Source: CAD feature listing. Evaluate the final solid. Frame: model axes, mm. A direction names the side the tool comes from. Round coordinates to 2 decimals unless told otherwise and drop trailing zeros. Loops run counter-clockwise (first coordinate to the right, second up) from the corner with the lowest first, then second, coordinate; pieces in that order, holes last.
(1) Mould query, pull axis X, two halves, no side actions, for faces 5 (the flat face through (17.635, -56, 0)), 6 (the cylindrical face through (-48.051, 12.783, 17.555)), 7 (the flat face through (-16, 28.78, 10)). Classes: pulls with the +X half, pulls with the -X half, needs draft (parallel to the pull), parting line crosses it, or undercut.
(2) Set-up query: faces 1 (the flat face through (-68.325, -38, 0)), 2 (the flat face through (-29, 23.82, 14)), 3 (the cylindrical face through (-59.61, 2.46, 0.05)), 4 (the flat face through (0.325, 26, 18)). Return all of +Z, -Z, +X, -X, +Y, -Y with unobstructed straight access to the full face (end or side cutting, diameter ignored); none if empty.
(3) First-contact query: pin 1 Ø17.5 at (x, y) = (-52.5, -55) entering from +Z; pin 2 Ø3 at (y, z) = (-63, 12) entering from -X (3 decimals); pin 3 Ø1.2 at (x, y) = (-38, 0.5) entering from +Z; pin 4 Ø13 at (x, y) = (-62.825, 0) entering from -Z. Flat tips, straight axial feed; report the tip coordinate or a pass-through.
(4) Material intervals for probe 1 along X at (y, z) = (0.5, 15.5); probe 2 along Y at (x, z) = (-10.5, 14.5); probe 3 along Z at (x, y) = (-48, 14), sorted ascending.
(5) Section D-D, the plane x = -14. Return the cut outline in (y, z).
(6) Section A-A, the plane y = -17.65. Return the cut outline in (x, z) (3 decimals), plus the area to 3 significant figures.
(7) Section C-C, the plane y = 20.78. Return the cut outline in (x, z) (3 decimals), plus the area to 3 significant figures.
(8) Section B-B, the plane z = 12. Return the cut outline in (x, y) (3 decimals), plus the area to 3 significant figures.
```python
from build123d import *

# Parameters (mm, degrees)
SALIENTE_EXTRUIR1_DEPTH    = 3.84
SALIENTE_EXTRUIR2_DEPTH    = 27.82
CROQUIS5_W                 = 19.2
CROQUIS5_H                 = 4.96
SALIENTE_EXTRUIR3_DEPTH    = 20.22
REDONDEO1_R                = 0.6
REDONDEO4_R                = 0.6
CROQUIS6_R                 = 2.36
CORTAR_EXTRUIR1_DEPTH      = 53.95
SALIENTE_EXTRUIR6_DEPTH    = 27.82
CORTAR_EXTRUIR9_DEPTH      = 53
CORTAR_EXTRUIR9_DEPTH_BACK = 66
CROQUIS10_R                = 2.36
REDONDEO5_R                = 5
REDONDEO6_R                = 5
CROQUIS12_R                = 4.05
CORTAR_EXTRUIR10_DEPTH     = 15
REDONDEO8_R                = 2
REDONDEO9_R                = 1
REDONDEO10_R               = 1
REDONDEO12_R               = 2
REDONDEO13_R               = 1
REDONDEO14_R               = 1
REDONDEO15_R               = 2
REDONDEO16_R               = 2
REDONDEO17_R               = 2
REDONDEO18_R               = 1
CROQUIS14_R                = 13.54
SALIENTE_EXTRUIR7_DEPTH    = 1
CROQUIS15_R                = 10.98
CORTAR_EXTRUIR12_DEPTH     = 4
CROQUIS16_R                = 4.05
CORTAR_EXTRUIR13_DEPTH     = 24
CROQUIS17_R                = 7.545
SALIENTE_EXTRUIR8_DEPTH    = 3
SALIENTE_EXTRUIR9_DEPTH    = 5
SALIENTE_EXTRUIR10_DEPTH   = 4
SALIENTE_EXTRUIR11_START   = 20
CROQUIS23_R                = 4.05
SALIENTE_EXTRUIR11_DEPTH   = 20
SALIENTE_EXTRUIR12_START   = 30
CROQUIS18_R                = 4.05
SALIENTE_EXTRUIR12_DEPTH   = 30
REDONDEO19_R               = 1.5
REDONDEO20_R               = 2
CROQUIS24_R                = 7.545
SALIENTE_EXTRUIR13_DEPTH   = 5
CROQUIS25_R                = 4.05
SALIENTE_EXTRUIR14_DEPTH   = 64
REDONDEO21_R               = 2


with BuildPart() as part:
    # Croquis1 → Saliente-Extruir1 (new, symmetric)
    with BuildSketch(Plane.XY):
        with BuildLine():
            Line((-68.325, 28.78), (68.325, 28.78))
            Line((68.325, 28.78), (68.325, -31.7))
            Line((68.325, -31.7), (35.165, -31.7))
            ThreePointArc((35.165, -31.7), (22.769418126, -36.834418126), (17.635, -49.23))
            Line((17.635, -49.23), (17.635, -64.4))
            Line((17.635, -64.4), (-68.325, -64.4))
            Line((-68.325, -64.4), (-68.325, -11.9))
            Line((-68.325, -11.9), (-73.325, -7.775))
            Line((-73.325, -7.775), (-73.325, 7.775))
            Line((-73.325, 7.775), (-68.325, 11.9))
            Line((-68.325, 11.9), (-68.325, 28.78))
        make_face()
    extrude(amount=SALIENTE_EXTRUIR1_DEPTH, both=True)

    # Croquis2 → Saliente-Extruir2 (add)
    with BuildSketch(Plane.XY.offset(3.84)):
        with BuildLine():
            Line((-58.075, 23.18), (-58.075, 28.78))
            Line((-58.075, 28.78), (-38.475, 28.78))
            Line((-38.475, 28.78), (-38.475, 23.18))
            ThreePointArc((-38.475, 23.18), (-48.275, 12.78), (-58.075, 23.18))
        make_face()
        with BuildLine():
            Line((-19.275, 23.18), (-19.275, 28.78))
            Line((-19.275, 28.78), (0.325, 28.78))
            Line((0.325, 28.78), (0.325, 23.18))
            ThreePointArc((0.325, 23.18), (-9.475, 12.78), (-19.275, 23.18))
        make_face()
    extrude(amount=SALIENTE_EXTRUIR2_DEPTH)

    # Croquis5 → Saliente-Extruir3 (add)
    with BuildSketch(Plane.XY.offset(3.84)):
        with Locations((-28.875, 26.3)):
            Rectangle(CROQUIS5_W, CROQUIS5_H)
    extrude(amount=SALIENTE_EXTRUIR3_DEPTH)

    # Redondeo1
    redondeo1_edges = [part.edges().sort_by_distance(p)[0] for p in [
        (-38.475, 23.82, 13.95),
    ]]
    fillet(redondeo1_edges, radius=REDONDEO1_R)

    # Redondeo4
    redondeo4_edges = [part.edges().sort_by_distance(p)[0] for p in [
        (-19.275, 23.82, 13.95),
    ]]
    fillet(redondeo4_edges, radius=REDONDEO4_R)

    # Croquis6 → Cortar-Extruir1 (cut, symmetric)
    with BuildSketch(Plane.XY):
        with Locations((-48.275, 20.78)):
            Circle(CROQUIS6_R)
        with Locations((-9.475, 20.78)):
            Circle(CROQUIS6_R)
    extrude(amount=CORTAR_EXTRUIR1_DEPTH, both=True, mode=Mode.SUBTRACT)

    # Croquis9 → Saliente-Extruir6 (add)
    with BuildSketch(Plane.XY.offset(3.84)):
        with BuildLine():
            Line((-58.075, -58.8), (-58.075, -64.4))
            Line((-58.075, -64.4), (-38.475, -64.4))
            Line((-38.475, -64.4), (-38.475, -58.8))
            ThreePointArc((-38.475, -58.8), (-48.275, -48.4), (-58.075, -58.8))
        make_face()
    extrude(amount=SALIENTE_EXTRUIR6_DEPTH)

    # Croquis10 → Cortar-Extruir9 (cut, two sides: drawn at the far end of the back side and taken through both)
    with BuildSketch(Plane.XY.offset(3.84).offset(-CORTAR_EXTRUIR9_DEPTH_BACK)):
        with Locations(Location((-48.275, -56.4, 0), (0, 0, 180))):
            Circle(CROQUIS10_R)
    extrude(amount=CORTAR_EXTRUIR9_DEPTH + CORTAR_EXTRUIR9_DEPTH_BACK, mode=Mode.SUBTRACT)

    # Redondeo5
    redondeo5_edges = [part.edges().sort_by_distance(p)[0] for p in [
        (-73.325, -7.775, 0),
    ]]
    fillet(redondeo5_edges, radius=REDONDEO5_R)

    # Redondeo6
    redondeo6_edges = [part.edges().sort_by_distance(p)[0] for p in [
        (-73.325, 7.775, 0),
    ]]
    fillet(redondeo6_edges, radius=REDONDEO6_R)

    # Croquis12 → Cortar-Extruir10 (cut, symmetric)
    with BuildSketch(Plane.XY.offset(3.84)):
        with Locations(Location((-62.825, 0, 0), (0, 0, 180))):
            Circle(CROQUIS12_R)
        with Locations(Location((-38.625, 0, 0), (0, 0, 180))):
            Circle(CROQUIS12_R)
    extrude(amount=CORTAR_EXTRUIR10_DEPTH, both=True, mode=Mode.SUBTRACT)

    # Redondeo8
    redondeo8_edges = [part.edges().sort_by_distance(p)[0] for p in [
        (-68.325, 28.78, 0),
    ]]
    fillet(redondeo8_edges, radius=REDONDEO8_R)

    # Redondeo9
    redondeo9_edges = [part.edges().sort_by_distance(p)[0] for p in [
        (-58.075, 28.78, 17.75),
    ]]
    fillet(redondeo9_edges, radius=REDONDEO9_R)

    # Redondeo10
    redondeo10_edges = [part.edges().sort_by_distance(p)[0] for p in [
        (-19.275, 28.78, 27.86),
    ]]
    fillet(redondeo10_edges, radius=REDONDEO10_R)

    # Redondeo12
    redondeo12_edges = [part.edges().sort_by_distance(p)[0] for p in [
        (-68.325, -64.4, 0),
    ]]
    fillet(redondeo12_edges, radius=REDONDEO12_R)

    # Redondeo13
    redondeo13_edges = [part.edges().sort_by_distance(p)[0] for p in [
        (-38.475, 28.78, 27.86),
    ]]
    fillet(redondeo13_edges, radius=REDONDEO13_R)

    # Redondeo14
    redondeo14_edges = [part.edges().sort_by_distance(p)[0] for p in [
        (0.325, 28.78, 17.75),
    ]]
    fillet(redondeo14_edges, radius=REDONDEO14_R)

    # Redondeo15
    redondeo15_edges = [part.edges().sort_by_distance(p)[0] for p in [
        (68.325, 28.78, 0),
    ]]
    fillet(redondeo15_edges, radius=REDONDEO15_R)

    # Redondeo16
    redondeo16_edges = [part.edges().sort_by_distance(p)[0] for p in [
        (68.325, -31.7, 0),
    ]]
    fillet(redondeo16_edges, radius=REDONDEO16_R)

    # Redondeo17
    redondeo17_edges = [part.edges().sort_by_distance(p)[0] for p in [
        (17.635, -64.4, 0),
    ]]
    fillet(redondeo17_edges, radius=REDONDEO17_R)

    # Redondeo18
    redondeo18_edges = [part.edges().sort_by_distance(p)[0] for p in [
        (-38.475, -64.4, 17.75),
    ]]
    fillet(redondeo18_edges, radius=REDONDEO18_R)

    # Croquis14 → Saliente-Extruir7 (add)
    with BuildSketch(Plane.XY.offset(3.84)):
        with Locations(Location((-32.475, -17.65, 0), (0, 0, 180))):
            Circle(CROQUIS14_R)
    extrude(amount=SALIENTE_EXTRUIR7_DEPTH)

    # Croquis15 → Cortar-Extruir12 (cut)
    with BuildSketch(Plane.XY.offset(4.84)):
        with Locations((-32.475, -17.65)):
            Circle(CROQUIS15_R)
    extrude(amount=-CORTAR_EXTRUIR12_DEPTH, mode=Mode.SUBTRACT)

    # Croquis16 → Cortar-Extruir13 (cut)
    with BuildSketch(Plane.XY.offset(0.84)):
        with Locations((-32.475, -17.65)):
            Circle(CROQUIS16_R)
    extrude(amount=-CORTAR_EXTRUIR13_DEPTH, mode=Mode.SUBTRACT)

    # Croquis17 → Saliente-Extruir8 (add)
    with BuildSketch(Plane.XY.offset(3.84)):
        with Locations(Location((-62.825, 0, 0), (0, 0, 180))):
            Circle(CROQUIS17_R)
    extrude(amount=SALIENTE_EXTRUIR8_DEPTH)

    # Croquis20 → Saliente-Extruir9 (add)
    with BuildSketch(Plane.XY.offset(3.84)):
        with BuildLine():
            ThreePointArc((-32.12244902, -4.114590593), (-41.156957864, 7.26651322), (-41.162580782, -7.264551519))
            ThreePointArc((-41.162580782, -7.264551519), (-36.930192915, -4.863958545), (-32.12244902, -4.114590593))
        make_face()
    extrude(amount=SALIENTE_EXTRUIR9_DEPTH)

    # Croquis22 → Saliente-Extruir10 (add)
    with BuildSketch(Plane.XY.offset(4.84)):
        with BuildLine():
            ThreePointArc((-41.158112573, -7.260815429), (-36.094687333, -7.261791639), (-32.128271446, -4.114440192))
            ThreePointArc((-32.128271446, -4.114440192), (-36.930192915, -4.863958545), (-41.158112573, -7.260815429))
        make_face()
    extrude(amount=SALIENTE_EXTRUIR10_DEPTH)

    # Croquis23 → Saliente-Extruir11 (add)
    with BuildSketch(Plane.XY.offset(8.84).offset(SALIENTE_EXTRUIR11_START)):
        with Locations(Location((-38.625, 0, 0), (0, 0, 180))):
            Circle(CROQUIS23_R)
    extrude(amount=-SALIENTE_EXTRUIR11_DEPTH)

    # Croquis18 → Saliente-Extruir12 (add)
    with BuildSketch(Plane.XY.offset(6.84).offset(SALIENTE_EXTRUIR12_START)):
        with Locations(Location((-62.825, 0, 0), (0, 0, 180))):
            Circle(CROQUIS18_R)
    extrude(amount=-SALIENTE_EXTRUIR12_DEPTH)

    # Redondeo19
    redondeo19_edges = [part.edges().sort_by_distance(p)[0] for p in [
        (-58.775, 0, 36.84),
    ]]
    fillet(redondeo19_edges, radius=REDONDEO19_R)

    # Redondeo20
    redondeo20_edges = [part.edges().sort_by_distance(p)[0] for p in [
        (-34.575, 0, 28.84),
    ]]
    fillet(redondeo20_edges, radius=REDONDEO20_R)

    # Croquis24 → Saliente-Extruir13 (add)
    with BuildSketch(Plane.XY.offset(3.84)):
        with Locations(Location((-8.283343025, -32.895909544, 0), (0, 0, 180))):
            Circle(CROQUIS24_R)
    extrude(amount=SALIENTE_EXTRUIR13_DEPTH)

    # Croquis25 → Saliente-Extruir14 (add)
    with BuildSketch(Plane.XY.offset(8.84)):
        with Locations((-8.283343025, -32.895909544)):
            Circle(CROQUIS25_R)
    extrude(amount=SALIENTE_EXTRUIR14_DEPTH)

    # Redondeo21
    redondeo21_edges = [part.edges().sort_by_distance(p)[0] for p in [
        (-12.333343025, -32.895909544, 72.84),
    ]]
    fillet(redondeo21_edges, radius=REDONDEO21_R)


solid = part.part
```
Output values:
1. face 5: pulls with the +X half
1. face 6: undercut
1. face 7: needs draft
2. face 1: +Z, -Z, -X, -Y
2. face 2: +Z
2. face 3: -Z
2. face 4: +Z, +X, +Y, -Y
3. pin 1: stops at z = 31.66
3. pin 2: stops at x = -58.075
3. pin 3: stops at z = 28.84
3. pin 4: stops at z = -3.84
4. probe 1: x = -66.84 to -58.81, -42.64 to -34.61
4. probe 2: y = -36.29 to -29.51, 12.83 to 18.65, 22.91 to 28.78
4. probe 3: z = -3.84 to 31.66
5. outline: (-64.4, -3.84) - (28.78, -3.84) - (28.78, 31.66) - (13.89, 31.66) - (13.89, 3.84) - (-27.97, 3.84) - (-27.97, 8.84) - (-37.82, 8.84) - (-37.82, 3.84) - (-64.4, 3.84) - close
6. outline: (-68.325, -3.84) - (-36.525, -3.84) - (-36.525, 0.84) - (-43.455, 0.84) - (-43.455, 4.84) - (-46.015, 4.84) - (-46.015, 3.84) - (-68.325, 3.84) - close; (-28.425, -3.84) - (68.325, -3.84) - (68.325, 3.84) - (-18.935, 3.84) - (-18.935, 4.84) - (-21.495, 4.84) - (-21.495, 0.84) - (-28.425, 0.84) - close
6. area: 951 mm2
7. outline: (-68.325, -3.84) - (-50.635, -3.84) - (-50.635, 31.66) - (-57.923, 31.66) - (-57.923, 3.84) - (-68.325, 3.84) - close; (-45.915, -3.84) - (-11.835, -3.84) - (-11.835, 31.66) - (-19.123, 31.66) - (-19.123, 3.84) - (-38.627, 3.84) - (-38.627, 31.66) - (-45.915, 31.66) - close; (-7.115, -3.84) - (68.325, -3.84) - (68.325, 3.84) - (0.173, 3.84) - (0.173, 31.66) - (-7.115, 31.66) - close
7. area: 1,790 mm2
8. outline: circle Ø8.1 at (-62.825, 0); (-58.075, -64.4) - (-39.475, -64.4) arc R1 ccw to (-38.475, -63.4) - (-38.475, -58.8) arc R9.817 ccw (long way) to (-58.075, -58.8) - close; (-58.075, 23.18) arc R9.817 ccw (long way) to (-38.475, 23.18) - (-38.475, 23.22) arc R0.6 cw to (-37.875, 23.82) - (-19.875, 23.82) arc R0.6 cw to (-19.275, 23.22) - (-19.275, 23.18) arc R9.817 ccw (long way) to (0.325, 23.18) - (0.325, 27.78) arc R1 ccw to (-0.675, 28.78) - (-57.075, 28.78) arc R1 ccw to (-58.075, 27.78) - close; circle Ø8.1 at (-38.625, 0); circle Ø8.1 at (-8.283, -32.896); hole circle Ø4.72 at (-48.275, -56.4); hole circle Ø4.72 at (-48.275, 20.78); hole circle Ø4.72 at (-9.475, 20.78)
8. area: 1,010 mm2
